from build123d import *

# Parameters (mm, degrees)
SKETCH1_W          = 23.368
SKETCH1_H          = 36.5125
SKETCH1_R          = 2.921
BASE_FLANGE1_DEPTH = 2.032
HEM1_START         = -18.25625
HEM1_DEPTH         = 36.5125
HEM1_2_DEPTH       = 36.5125
CHAMFER1_SIZE      = 1.016


# Read off the part's stored shape, not the designer's step: Hem1
# Sheet-metal steps are written as plain solids
with BuildPart() as part:
    # Sketch1 → Base-Flange1 (new body)
    with BuildSketch(Plane(origin=(0, 0, 0), x_dir=(1, 0, 0), z_dir=(0, 1, 0))):
        Rectangle(SKETCH1_W, SKETCH1_H)
        with Locations(Location((-4.064, -11.1125, 0), (0, 0, 270))):
            Circle(SKETCH1_R, mode=Mode.SUBTRACT)
        with Locations(Location((-4.064, 11.1125, 0), (0, 0, 270))):
            Circle(SKETCH1_R, mode=Mode.SUBTRACT)
    extrude(amount=BASE_FLANGE1_DEPTH)

    # Hem1 outline → Hem1 (cut)
    with BuildSketch(Plane.XY.offset(HEM1_START)):
        with BuildLine():
            Line((11.684, 2.032), (11.139527241, 2.032))
            ThreePointArc((11.139527241, 2.032), (9.652, 0.544472759), (7.62, 0))
            Line((7.62, 0), (11.684, 0))
            Line((11.684, 0), (11.684, 2.032))
        make_face()
    extrude(amount=HEM1_DEPTH, mode=Mode.SUBTRACT)

    # Hem1 2 outline → Hem1 2 (add)
    with BuildSketch(Plane.XY.offset(HEM1_START)):
        with BuildLine():
            Line((3.801089189, 2.674030138), (5.710544595, 3.369015069))
            ThreePointArc((5.710544595, 3.369015069), (8.785507319, 5.728516954), (7.62, 2.032))
            Line((7.62, 2.032), (11.139527241, 2.032))
            ThreePointArc((11.139527241, 2.032), (7.974200939, 8.112535253), (3.801089189, 2.674030138))
        make_face()
    extrude(amount=HEM1_2_DEPTH)

    # Chamfer1
    chamfer1_edges = [part.edges().sort_by_distance(p)[0] for p in [
        (-4.064, 2.032, 8.1915),
        (-4.064, 2.032, -14.0335),
    ]]
    chamfer(chamfer1_edges, length=CHAMFER1_SIZE)


solid = part.part
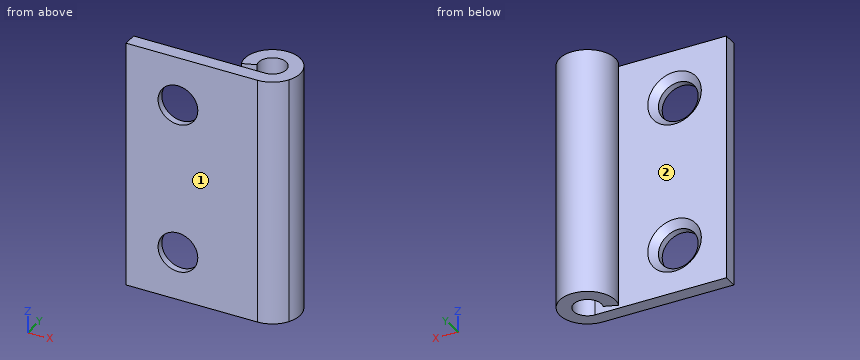
Could you check a few things on this model? Use its own coordinates, in mm. Face numbers are marked on the shaded views. A direction names the side the tool comes from. Give positions to 0.01 mm unless a question says otherwise; leave off trailing zeros. Order: outer loops, then holes, each group sorted by start corner. A loop starts at its lowest first (then second) coordinate and runs counter-clockwise, first axis right, second up. Notation, with made-up numbers: (-19, 23) - (17, 23) arc R26 ccw to (17, 45) - close; hole circle Ø9 at (82.25, -1.5). An arc over 180 degrees is marked (long way). Return JSON: item names as keys, results as strings. Group by question number.
Q1. Will these pins go through, and if not, where does the flat tip stop? pin 1 Ø6 at (x, z) = (-0.5, 4) entering from +Y; pin 2 Ø3.5 at (x, z) = (-4.06, 11.11) entering from -Y; pin 3 Ø3 at (x, z) = (4, 9) entering from +Y.
Q2. Suppose I cut it at D-D, the plane y = 7.5. Please give me the cut outline in (x, z).
Q3. Suppose I cut it at B-B, the plane z = 16.5. Please give me the cut outline in (x, y), and give its area (3 significant figures).
Q4. Which directions (+Z, -Z, +X, -X, +Y, -Y) give clear straight access to the entire face, cutting with the end or side of a thin tool? Please do the marked faces 1 and 2.
Q5. Suppose I cut it at C-C, the plane x = 0.5. Please give me the cut outline in (y, z).
Q6. Please list where these lines run through material, in increasing order: line 1 along Z through (x, y) = (-5, 1.5); line 2 along Y through (x, z) = (0.5, 12); line 3 along X through (y, z) = (3.75, 2). Write a range as [from, to].
Q7. Suppose I cut it at A-A, the plane y = 5.5. Please give me the cut outline in (x, z), and give its area (3 significant figures).
Resolved:
{
 "1": {"pin 1": "stops at y = 2.03", "pin 2": "passes through", "pin 3": "stops at y = 7.53"},
 "2": {"outline": "(5.45, -18.26) - (9.79, -18.26) - (9.79, 18.26) - (5.45, 18.26) - close"},
 "3": {"outline": "(-11.68, 0) - (7.62, 0) arc R4.06 ccw (long way) to (3.8, 2.67) - (5.71, 3.37) arc R2.03 cw (long way) to (7.62, 2.03) - (-11.68, 2.03) - close", "area": "70.6 mm2"},
 "4": {"face 1": "+Z, -Z, +X, -X, -Y", "face 2": "+Z, -Z, -X"},
 "5": {"outline": "(0, -18.26) - (2.03, -18.26) - (2.03, 18.26) - (0, 18.26) - close"},
 "6": {"line 1": "z = [-18.26, -14.39], [-7.84, 7.84], [14.39, 18.26]", "line 2": "y = [0, 2.03]", "line 3": "x = [3.57, 5.61], [9.63, 11.67]"},
 "7": {"outline": "(3.82, -18.26) - (6.18, -18.26) - (6.18, 18.26) - (3.82, 18.26) - close; (9.06, -18.26) - (11.42, -18.26) - (11.42, 18.26) - (9.06, 18.26) - close", "area": "173 mm2"}
}
